```python
from build123d import *

# Parameters (mm, degrees)
BOSS_EXTRUDE1_DEPTH = 55
SKETCH5_R           = 5
CUT_EXTRUDE2_DEPTH  = 9.89


with BuildPart() as part:
    # Sketch1 → Boss-Extrude1 (new body, symmetric)
    with BuildSketch(Plane(origin=(0, 0, 0), x_dir=(1, 0, 0), z_dir=(0, 1, 0))):
        with BuildLine():
            Line((-38.1, -3.4925), (-38.1, -3.81))
            Line((-38.1, -3.81), (-34.739896, -3.81))
            ThreePointArc((-34.739896, -3.81), (-33.469896, -2.090104), (-33.02, 0))
            ThreePointArc((-33.02, 0), (-33.469896, 2.090104), (-34.739896, 3.81))
            Line((-34.739896, 3.81), (-38.1, 3.81))
            Line((-38.1, 3.81), (-38.1, 3.4925))
            ThreePointArc((-38.1, 3.4925), (-35.63043, 2.46957), (-34.6075, 0))
            ThreePointArc((-34.6075, 0), (-35.63043, -2.46957), (-38.1, -3.4925))
        make_face()
        with BuildLine():
            Line((-34.739896, -3.81), (-38.1, -3.81))
            Line((-38.1, -3.81), (-38.1, -3.4925))
            ThreePointArc((-38.1, -3.4925), (-41.5925, 0), (-38.1, 3.4925))
            Line((-38.1, 3.4925), (-38.1, 3.81))
            Line((-38.1, 3.81), (-34.739896, 3.81))
            ThreePointArc((-34.739896, 3.81), (-43.18, 0), (-34.739896, -3.81))
        make_face()
        with BuildLine():
            ThreePointArc((-33.02, 0), (-33.469896, -2.090104), (-34.739896, -3.81))
            Line((-34.739896, -3.81), (34.739896, -3.81))
            ThreePointArc((34.739896, -3.81), (33.02, 0), (34.739896, 3.81))
            Line((34.739896, 3.81), (-34.739896, 3.81))
            ThreePointArc((-34.739896, 3.81), (-33.469896, 2.090104), (-33.02, 0))
        make_face()
        with BuildLine():
            ThreePointArc((34.739896, 3.81), (33.02, 0), (34.739896, -3.81))
            Line((34.739896, -3.81), (38.1, -3.81))
            Line((38.1, -3.81), (38.1, -3.4925))
            ThreePointArc((38.1, -3.4925), (34.6075, 0), (38.1, 3.4925))
            Line((38.1, 3.4925), (38.1, 3.81))
            Line((38.1, 3.81), (34.739896, 3.81))
        make_face()
        with BuildLine():
            Line((38.1, -3.81), (34.739896, -3.81))
            ThreePointArc((34.739896, -3.81), (40.190104, -4.630104), (43.18, 0))
            ThreePointArc((43.18, 0), (40.190104, 4.630104), (34.739896, 3.81))
            Line((34.739896, 3.81), (38.1, 3.81))
            Line((38.1, 3.81), (38.1, 3.4925))
            ThreePointArc((38.1, 3.4925), (40.56957, 2.46957), (41.5925, 0))
            ThreePointArc((41.5925, 0), (40.56957, -2.46957), (38.1, -3.4925))
            Line((38.1, -3.4925), (38.1, -3.81))
        make_face()
    extrude(amount=BOSS_EXTRUDE1_DEPTH, both=True)

    # Sketch5 → Cut-Extrude2 (cut, through all)
    with BuildSketch(Plane.XY.offset(3.81)):
        with Locations((-25.260104, -48)):
            Circle(SKETCH5_R)
        with Locations((-25.260104, -23)):
            Circle(SKETCH5_R)
        with Locations((4.739896, 47)):
            Circle(SKETCH5_R)
        with Locations((4.739896, -45)):
            Circle(SKETCH5_R)
        with Locations((24.739896, 1)):
            Circle(SKETCH5_R)
        with Locations((-25.260104, 27)):
            Circle(SKETCH5_R)
        with Locations((24.739896, 27)):
            Circle(SKETCH5_R)
        with Locations((-25.260104, -6.5)):
            Circle(SKETCH5_R)
        with Locations((4.739896, 7)):
            Circle(SKETCH5_R)
    extrude(amount=-CUT_EXTRUDE2_DEPTH, mode=Mode.SUBTRACT)


solid = part.part
```
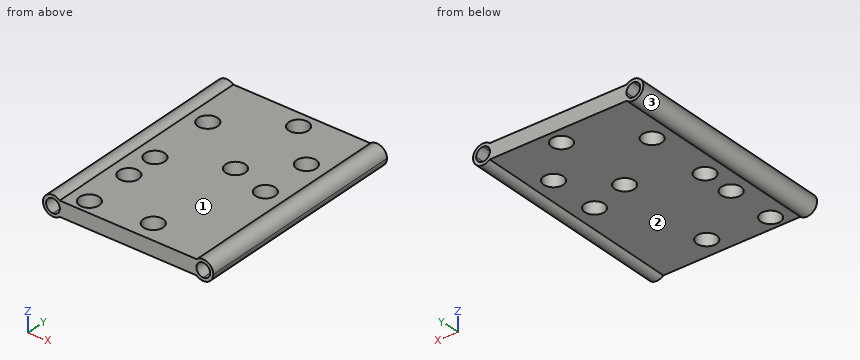
The model under review builds one solid part; all positions refer to its coordinate system, in mm. Face numbers are marked on the shaded views. A direction names the side the tool comes from. Coordinates: 2 decimals unless noted, no trailing zeros. Write each loop counter-clockwise with the first axis right and the second up, starting at its lowest first coordinate (ties: lowest second). Pieces come first, ordered by that corner, then holes.
1) We need section B-B on y = -23. State the section outline as (x, z) points (1 decimal), then the cut area to 3 significant figures.
2) Clearance check with flat-ended pins moving along their axes: pin 1 Ø16 at (x, y) = (4.74, 47) entering from -Z; pin 2 Ø3 at (y, z) = (-23, -2.5) entering from -X; pin 3 Ø4 at (y, z) = (-17.5, 2.5) entering from +X. State where each tip first meets the part, or that it passes through.
3) We need section D-D on y = -38. State the section outline as (x, z) points (1 decimal), then the cut area to 3 significant figures.
4) To check wall thickness, follow probe 1 along Y at (x, z) = (-25, 2.5); probe 2 along X at (y, z) = (-34, 0.25); probe 3 along X at (y, z) = (7.5, -2.5). State the ranges of each line that lie inside material, in increasing order.
5) We need section A-A on y = 27. State the section outline as (x, z) points (1 decimal), then the cut area to 3 significant figures.
6) We need section C-C on z = -1.5. Count the separate pieces of the cut face and the enclosed holes in it, then the cut area to 3 significant figures.
7) Machinability: for the marked faces 1, 2 and 3, which of the approach directions +Z, -Z, +X, -X, +Y, -Y give a long, thin tool a straight path to every point of the face, cutting with its end or side? Answer none if there is none.
Answer list:
1. outline: (-34.7, -3.8) - (-30.3, -3.8) - (-30.3, 3.8) - (-34.7, 3.8) arc R5.1 ccw (long way) to start; (-20.3, -3.8) - (34.7, -3.8) arc R5.1 ccw (long way) to (34.7, 3.8) - (-20.3, 3.8) - close; hole (-38.1, -3.5) arc R3.5 ccw to (-34.6, 0) arc R3.5 ccw to (-38.1, 3.5) arc R3.5 ccw to start; hole (38.1, -3.5) arc R3.5 ccw to (41.6, 0) arc R3.5 ccw to (38.1, 3.5) arc R3.5 ccw to start
1. area: 521 mm2
2. pin 1: stops at z = -3.81
2. pin 2: stops at x = -43.08
2. pin 3: stops at x = 43.16
3. outline: (-34.7, -3.8) - (34.7, -3.8) arc R5.1 ccw (long way) to (34.7, 3.8) - (-34.7, 3.8) arc R5.1 ccw (long way) to start; hole (-38.1, -3.5) arc R3.5 ccw to (-34.6, 0) arc R3.5 ccw to (-38.1, 3.5) arc R3.5 ccw to start; hole (38.1, -3.5) arc R3.5 ccw to (41.6, 0) arc R3.5 ccw to (38.1, 3.5) arc R3.5 ccw to start
3. area: 597 mm2
4. probe 1: y = -55 to -52.99, -43.01 to -27.99, -18.01 to -11.49, -1.51 to 22.01, 31.99 to 55
4. probe 2: x = -43.17 to -41.58, -34.62 to 34.62, 41.58 to 43.17
4. probe 3: x = -42.52 to -40.54, -35.66 to -0.24, 9.71 to 35.66, 40.54 to 42.52
5. outline: (-34.7, -3.8) - (-30.3, -3.8) - (-30.3, 3.8) - (-34.7, 3.8) arc R5.1 ccw (long way) to start; (-20.3, -3.8) - (19.7, -3.8) - (19.7, 3.8) - (-20.3, 3.8) - close; (29.7, -3.8) - (34.7, -3.8) arc R5.1 ccw (long way) to (34.7, 3.8) - (29.7, 3.8) - close; hole (-38.1, -3.5) arc R3.5 ccw to (-34.6, 0) arc R3.5 ccw to (-38.1, 3.5) arc R3.5 ccw to start; hole (38.1, -3.5) arc R3.5 ccw to (41.6, 0) arc R3.5 ccw to (38.1, 3.5) arc R3.5 ccw to start
5. area: 444 mm2
6. separate pieces: 3
6. enclosed holes: 9
6. area: 7,360 mm2
7. face 1: +Z, +Y, -Y
7. face 2: -Z, +Y, -Y
7. face 3: +Y, -Y
